Check sheet for the drawn part. Datum: minimum x, y, z corner. Units: mm. A direction names the side the tool comes from. Give positions to 0.01 mm unless a question says otherwise; leave off trailing zeros. Write each loop counter-clockwise with the first axis right and the second up, starting at its lowest first coordinate (ties: lowest second). Pieces come first, ordered by that corner, then holes.
(1) Tool access check on the marked faces 5, 6, 7, 8 and 9. Record the directions out of +Z, -Z, +X, -X, +Y, -Y that give a thin tool (end or side, any length) a straight path to the whole face; none if there is none.
(2) Thickness scan on line 1 along Y through (x, z) = (37.45, 2.5); line 2 along Y through (x, z) = (22, 1.7); line 3 along Y through (x, z) = (38.15, 2.5). Record the ranges inside material, lowest first.
(3) Depth check by flat-ended pin: P1, Ø1.2, axis at y = 18, z = 3.5, coming from the +X side; P2, Ø0.8, axis at x = 2.5, z = 1.5, coming from the +Y side; P3, Ø5.5, axis at x = 42, y = 16, coming from the +Z side. Enter the tip coordinate at first touch or a pass-through.
(4) Mould release check, pull along X, two halves, no side actions. Record for the marked faces 1, 2, 3 and 4: +X half, -X half, draft (parallel to the pull), parting line (faces both ways), or undercut.
(5) Cross-section at B-B (x = 22). Record the boundary of the cut face in (y, z).
(6) Cross-section at D-D (y = 25.5). Record the boundary of the cut face in (x, z).
(7) Cross-section at A-A (y = 16). Record the boundary of the cut face in (x, z), and give its area (3 significant figures).
(8) Cross-section at C-C (z = 4.3). Record the boundary of the cut face in (x, y), and give its area (3 significant figures).
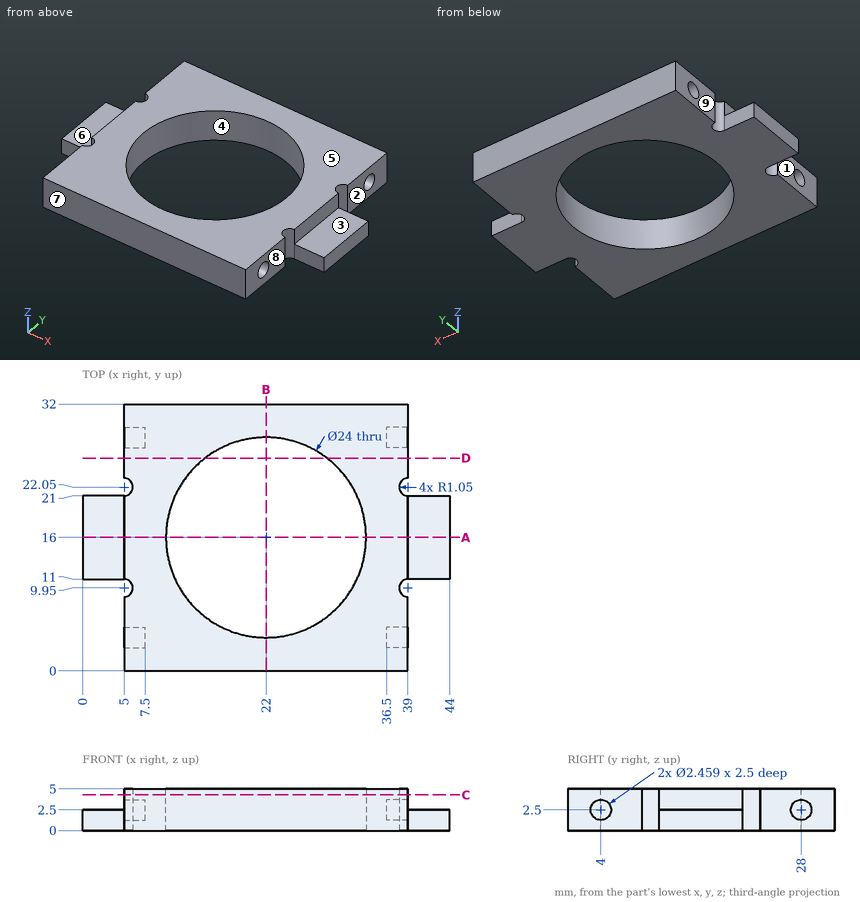
Reply:
1. face 5: +Z, +X, -X, +Y, -Y
1. face 6: +Z, -X, +Y, -Y
1. face 7: +Z, -Z, +X, -X, -Y
1. face 8: +Z, -Z, +X, -Y
1. face 9: +Z, -Z, -X, +Y
2. line 1: y = 0 to 2.77, 5.23 to 26.77, 29.23 to 32
2. line 2: y = 0 to 4, 28 to 32
2. line 3: y = 0 to 2.77, 5.23 to 9.33, 10.57 to 21.43, 22.67 to 26.77, 29.23 to 32
3. P1: stops at x = 39
3. P2: stops at y = 21
3. P3: stops at z = 2.5
4. face 1: -X half
4. face 2: +X half
4. face 3: draft
4. face 4: undercut
5. outline: (0, 0) - (4, 0) - (4, 5) - (0, 5) - close; (28, 0) - (32, 0) - (32, 5) - (28, 5) - close
6. outline: (5, 0) - (14.67, 0) - (14.67, 5) - (5, 5) - close; (29.33, 0) - (39, 0) - (39, 5) - (29.33, 5) - close
7. outline: (0, 0) - (10, 0) - (10, 5) - (5, 5) - (5, 2.5) - (0, 2.5) - close; (34, 0) - (44, 0) - (44, 2.5) - (39, 2.5) - (39, 5) - (34, 5) - close
7. area: 75.0 mm2
8. outline: (5, 0) - (39, 0) - (39, 8.9) arc R1.05 cw to (39, 11) - (39, 21) arc R1.05 cw to (39, 23.1) - (39, 32) - (5, 32) - (5, 23.1) arc R1.05 cw to (5, 21) - (5, 11) arc R1.05 cw to (5, 8.9) - close; hole circle Ø24 at (22, 16)
8. area: 629 mm2
